Build history of the part. All positions in model axes, mm. Face numbers are marked on the shaded views. Give positions to 0.01 mm unless a question says otherwise; leave off trailing zeros. Order: outer loops, then holes, each group sorted by start corner. A loop starts at its lowest first (then second) coordinate and runs counter-clockwise, first axis right, second up. Notation, with made-up numbers: (40.5, 18) - (94.5, 18) arc R13 ccw to (94.5, 31) - close; hole circle Ø10 at (19, 85.5). An arc over 180 degrees is marked (long way). Use a Markdown table: item, result.
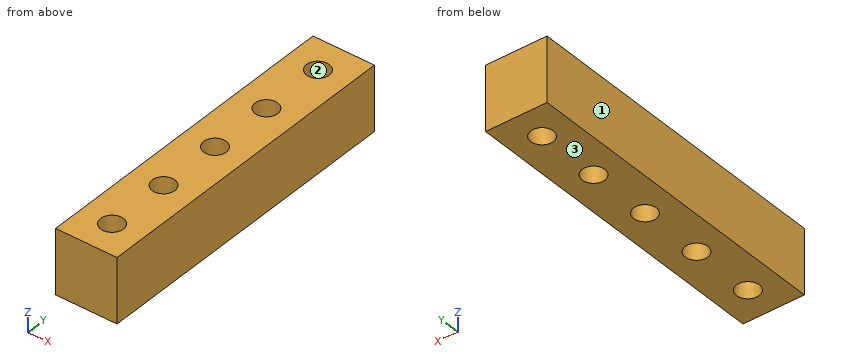
Autodesk Inventor part; units mm, degrees
ref_plane "YZ Plane" through (0, 0, 0) normal (1, 0, 0) x (0, 1, 0)
ref_plane "XZ Plane" through (0, 0, 0) normal (0, 1, 0) x (-1, 0, 0)
ref_plane "XY Plane" through (0, 0, 0) normal (0, 0, 1) x (1, 0, 0)
sketch "Sketch1" plane through (0, 0, 0) normal (0, 0, 1) x (1, 0, 0)
  line L0 (0, 0) -> (2.413, 0)
  line L1 (2.413, 0) -> (2.413, 12.7)
  line L2 (2.413, 12.7) -> (0, 12.7)
  line L3 (0, 12.7) -> (0, 0)
  circle A0 centre (1.2065, 11.43) radius 0.4445
  circle A1 centre (1.2065, 8.89) radius 0.4445
  circle A2 centre (1.2065, 6.35) radius 0.4445
  circle A3 centre (1.2065, 3.81) radius 0.4445
  circle A4 centre (1.2065, 1.27) radius 0.4445
  dimension "d0" = 2.413
  dimension "d1" = 12.7
  dimension "d2" = 0.889
  dimension "d3" = 0.889
  dimension "d4" = 0.889
  dimension "d5" = 1.27
  dimension "d6" = 2.54
  dimension "d7" = 2.54
  dimension "d8" = 0.889
  dimension "d9" = 0.889
  dimension "d10" = 2.54
  dimension "d11" = 2.54
  dimension "d12" = 1.2065
extrude "Extrusion1" add sketch "Sketch1" along normal blind 2.54
equation "\"d12\" = 0.5 * d0"
properties part number "5 pin header"
1) Slice it at C-C (y = 1). Write the cut outline in (x, z), and give its area (3 significant figures).
Computed:
| item | result |
|---|---|
| outline | (0, 0) - (0.85, 0) - (0.85, 2.54) - (0, 2.54) - close; (1.56, 0) - (2.41, 0) - (2.41, 2.54) - (1.56, 2.54) - close |
| area | 4.34 mm² |
2) Two-plate mould, pull along X, no slides. Class the marked faces 1, 2 and 3: +X half, -X half, draft (parallel to the pull), parting line (faces both ways), or undercut.
Computed:
| item | result |
|---|---|
| face 1 | -X half |
| face 2 | undercut |
| face 3 | draft |
3) Slice it at A-A (y = 8.89). Write the cut outline in (x, z).
Computed:
| item | result |
|---|---|
| outline | (0, 0) - (0.76, 0) - (0.76, 2.54) - (0, 2.54) - close; (1.65, 0) - (2.41, 0) - (2.41, 2.54) - (1.65, 2.54) - close |
4) Wall check: line 1 (Y direction, x = 1.35, z = 1.35); line 2 (Y direction, x = 0.9, z = 1.15); line 3 (X direction, y = 1.5, z = 1.85). Give the ranges that are in metal, low to high. Write a range as from..to.
Computed:
| item | result |
|---|---|
| line 1 | y = 0..0.85, 1.69..3.39, 4.23..5.93, 6.77..8.47, 9.31..11.01, 11.85..12.7 |
| line 2 | y = 0..0.95, 1.59..3.49, 4.13..6.03, 6.67..8.57, 9.21..11.11, 11.75..12.7 |
| line 3 | x = 0..0.83, 1.59..2.41 |
5) Slice it at B-B (z = 2.1). Write the cut outline in (x, y), and give its area (3 significant figures).
Computed:
| item | result |
|---|---|
| outline | (0, 0) - (2.41, 0) - (2.41, 12.7) - (0, 12.7) - close; hole circle Ø0.89 at (1.21, 1.27); hole circle Ø0.89 at (1.21, 3.81); hole circle Ø0.89 at (1.21, 6.35); hole circle Ø0.89 at (1.21, 8.89); hole circle Ø0.89 at (1.21, 11.43) |
| area | 27.5 mm² |
